Check sheet for the modelled part. Datum: model origin and axes. Units: mm. Face numbers are marked on the shaded views. A direction names the side the tool comes from. Coordinates: 2 decimals unless noted, no trailing zeros. Order: outer loops, then holes, each group sorted by start corner. A loop starts at its lowest first (then second) coordinate and runs counter-clockwise, first axis right, second up.
1. Cross-section at C-C (z = -32.5). Enter the section's corners in (x, y), then the cut area to 3 significant figures.
2. Thickness scan on line 1 (Y direction, x = 35.5, z = 2.8); line 2 (X direction, y = 220, z = 2); line 3 (X direction, y = 67, z = -23). Record the ranges inside material, lowest first.
3. Set-up check for the marked faces 1, 2, 3 and 4: record each of +Z, -Z, +X, -X, +Y, -Y from which the full face is reachable in a straight line by a thin tool's end or side.
4. Gauge pin test, flat ends, axial feed: pin 1 Ø3 at (y, z) = (187.5, -21.5) entering from -X; pin 2 Ø4 at (y, z) = (164, -6) entering from -X; pin 3 Ø12 at (x, y) = (2.5, 166.5) entering from -Z. Record the tip position at first contact, or that the pin passes through.
5. Draft check along X on the marked faces 5, 6 and 7. Enter one of: released by +X, released by -X, zero draft, split by the parting line, or undercut.
6. Cross-section at B-B (y = 86.5). Enter the section's corners in (x, z).
7. Cross-section at A-A (z = -20). Enter the section's corners in (x, y).
```python
from build123d import *

# Parameters (mm, degrees)
SKETCH1_W            = 111
SKETCH1_H            = 240
BOSS_EXTRUDE1_DEPTH  = 5
FILLET1_R            = 20
SKETCH2_R            = 4.25
BOSS_EXTRUDE2_DEPTH  = 10
FILLET2_R            = 8
FILLET3_R            = 5
FILLET2_OF_MIRROR1_R = 8
FILLET3_OF_MIRROR1_R = 5
SKETCH3_R            = 3.25
CUT_EXTRUDE1_DEPTH   = 250.560113109
SKETCH4_R            = 8
CUT_EXTRUDE2_DEPTH   = 250.560113109


with BuildPart() as part:
    # Sketch1 → Boss-Extrude1 (new body)
    with BuildSketch(Plane.XY):
        with Locations((0, 120)):
            Rectangle(SKETCH1_W, SKETCH1_H)
    extrude(amount=BOSS_EXTRUDE1_DEPTH)

    # Fillet1
    fillet1_edges = [part.edges().sort_by_distance(p)[0] for p in [
        (-55.5, 240, 2.5),
        (55.5, 240, 2.5),
        (55.5, 0, 2.5),
        (-55.5, 0, 2.5),
    ]]
    fillet(fillet1_edges, radius=FILLET1_R)

    # Sketch2 → Boss-Extrude2 (add)
    with BuildSketch(Plane(origin=(10.5, 0, 0), x_dir=(0, 0, -1), z_dir=(1, 0, 0))):
        with BuildLine():
            Line((0, 0), (30, 0))
            ThreePointArc((30, 0), (37.071067812, 2.928932188), (40, 10))
            Line((40, 10), (40, 200.857864376))
            ThreePointArc((40, 200.857864376), (39.238795325, 204.6846987), (37.071067812, 207.928932188))
            Line((37.071067812, 207.928932188), (7.928932188, 237.071067812))
            ThreePointArc((7.928932188, 237.071067812), (4.6846987, 239.238795325), (0.857864376, 240))
            Line((0.857864376, 240), (0, 240))
            Line((0, 240), (0, 0))
        make_face()
        with Locations((20, 190)):
            Circle(SKETCH2_R, mode=Mode.SUBTRACT)
        with Locations((20, 20)):
            Circle(SKETCH2_R, mode=Mode.SUBTRACT)
    boss_extrude2 = extrude(amount=BOSS_EXTRUDE2_DEPTH)

    # Fillet2
    fillet2_edges = [part.edges().sort_by_distance(p)[0] for p in [
        (20.5, 120, 0),
    ]]
    fillet(fillet2_edges, radius=FILLET2_R)

    # Fillet3
    fillet3_edges = [part.edges().sort_by_distance(p)[0] for p in [
        (10.5, 120, 0),
    ]]
    fillet(fillet3_edges, radius=FILLET3_R)

    # Mirror1: Boss-Extrude2 across plane
    add(boss_extrude2.mirror(Plane(origin=(0, 0, 0), x_dir=(0, 0, 1), z_dir=(1, 0, 0))))

    # Fillet2 of Mirror1
    fillet2_of_mirror1_edges = [part.edges().sort_by_distance(p)[0] for p in [
        (-20.5, 120, 0),
    ]]
    fillet(fillet2_of_mirror1_edges, radius=FILLET2_OF_MIRROR1_R)

    # Fillet3 of Mirror1
    fillet3_of_mirror1_edges = [part.edges().sort_by_distance(p)[0] for p in [
        (-10.5, 120, 0),
    ]]
    fillet(fillet3_of_mirror1_edges, radius=FILLET3_OF_MIRROR1_R)

    # Sketch3 → Cut-Extrude1 (cut, through all)
    with BuildSketch(Plane(origin=(0, 0, 0), x_dir=(-1, 0, 0), z_dir=(0, 0, -1))):
        with Locations((-35.5, 220)):
            Circle(SKETCH3_R)
        with Locations((-35.5, 20)):
            Circle(SKETCH3_R)
        with Locations((35.5, 20)):
            Circle(SKETCH3_R)
        with Locations((35.5, 220)):
            Circle(SKETCH3_R)
    extrude(amount=-CUT_EXTRUDE1_DEPTH, mode=Mode.SUBTRACT)

    # Sketch4 → Cut-Extrude2 (cut, through all)
    with BuildSketch(Plane(origin=(0, 0, 0), x_dir=(-1, 0, 0), z_dir=(0, 0, -1))):
        with Locations((-35.5, 220)):
            Circle(SKETCH4_R)
        with Locations((35.5, 220)):
            Circle(SKETCH4_R)
        with Locations((35.5, 20)):
            Circle(SKETCH4_R)
        with Locations((-35.5, 20)):
            Circle(SKETCH4_R)
    extrude(amount=CUT_EXTRUDE2_DEPTH, mode=Mode.SUBTRACT)


solid = part.part
```
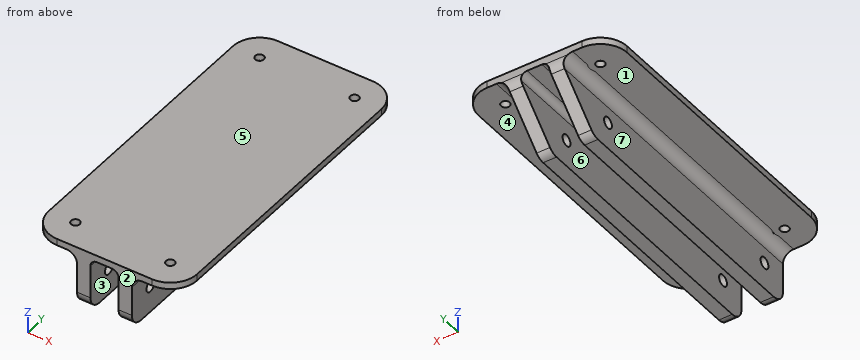
Data:
1. outline: (-20.5, 0.32) - (-10.5, 0.32) - (-10.5, 212.5) - (-20.5, 212.5) - close; (10.5, 0.32) - (20.5, 0.32) - (20.5, 212.5) - (10.5, 212.5) - close
1. area: 4,240 mm2
2. line 1: y = 0 to 16.75, 23.25 to 216.75, 223.25 to 240
2. line 2: x = -55.5 to -38.75, -32.25 to 32.25, 38.75 to 55.5
2. line 3: x = -20.5 to -10.5, 10.5 to 20.5
3. face 1: -Z, -X, +Y, -Y
3. face 2: +Z, -Z, +X, -X, -Y
3. face 3: -Z, +Y, -Y
3. face 4: -Z, +X, +Y, -Y
4. pin 1: stops at x = -20.5
4. pin 2: stops at x = -21.57
4. pin 3: stops at z = -1
5. face 5: zero draft
5. face 6: undercut
5. face 7: released by -X
6. outline: (-55.5, 0) - (-28.5, 0) arc R8 cw to (-20.5, -8) - (-20.5, -40) - (-10.5, -40) - (-10.5, -5) arc R5 cw to (-5.5, 0) - (5.5, 0) arc R5 cw to (10.5, -5) - (10.5, -40) - (20.5, -40) - (20.5, -8) arc R8 cw to (28.5, 0) - (55.5, 0) - (55.5, 5) - (-55.5, 5) - close
7. outline: (-20.5, 0) - (-10.5, 0) - (-10.5, 15.75) - (-20.5, 15.75) - close; (-20.5, 24.25) - (-10.5, 24.25) - (-10.5, 185.75) - (-20.5, 185.75) - close; (-20.5, 194.25) - (-10.5, 194.25) - (-10.5, 225) - (-20.5, 225) - close; (10.5, 0) - (20.5, 0) - (20.5, 15.75) - (10.5, 15.75) - close; (10.5, 24.25) - (20.5, 24.25) - (20.5, 185.75) - (10.5, 185.75) - close; (10.5, 194.25) - (20.5, 194.25) - (20.5, 225) - (10.5, 225) - close
